Can you work these out from the model? Positions are in its coordinate system, mm. A direction names the side the tool comes from. Coordinates: 2 decimals unless noted, no trailing zeros. Write each loop counter-clockwise with the first axis right and the second up, starting at its lowest first coordinate (ties: lowest second). Pieces come first, ordered by that corner, then holes. Notation, with made-up numbers: M 80,-5.5 L 118,-5.5 A26 ccw 118,29.5 Z; hole C 40.5,85 d11. An arc over 180 degrees is marked long. Answer as a JSON object with one key per item and string values. Group by question number.
from build123d import *

# Parameters (mm, degrees)
SKETCH1_R                = 15
BOSS_EXTRUDE1_DEPTH      = 75
CUT_EXTRUDE1_DEPTH       = 52
CUT_EXTRUDE2_DEPTH       = 3.5
SKETCH9_R                = 10
CUT_EXTRUDE12_DEPTH      = 70
SKETCH17_W               = 7
SKETCH17_H               = 12
CUT_EXTRUDE19_DEPTH      = 15
SKETCH19_W               = 7
SKETCH19_H               = 12
CUT_EXTRUDE20_DEPTH      = 15
SKETCH20_R               = 7.5
CUT_EXTRUDE21_DEPTH      = 40
CUT_EXTRUDE25_DEPTH      = 152.492574075
CUT_EXTRUDE25_DEPTH_BACK = 55
SKETCH21_W               = 20
SKETCH21_H               = 7.639320226
CUT_EXTRUDE28_DEPTH      = 152.492574075
CUT_EXTRUDE28_DEPTH_BACK = 10
SKETCH24_R               = 15
SKETCH25_R               = 15
CUT_EXTRUDE29_DEPTH      = 10
CUT_EXTRUDE30_DEPTH      = 81.841883926
CUT_EXTRUDE30_DEPTH_BACK = 81.841883926


with BuildPart() as part:
    # Sketch1 → Boss-Extrude1 (new, symmetric)
    with BuildSketch(Plane(origin=(0, 0, 0), x_dir=(1, 0, 0), z_dir=(0, 1, 0))):
        with Locations(Location((0, 0, 0), (0, 0, 270))):
            Circle(SKETCH1_R)
    extrude(amount=BOSS_EXTRUDE1_DEPTH, both=True)

    # Sketch2 → Cut-Extrude1 (cut)
    with BuildSketch(Plane.XZ.offset(75)):
        with BuildLine():
            Line((3.5, 15), (3.5, -15))
            ThreePointArc((3.5, -15), (0, -18.5), (-3.5, -15))
            Line((-3.5, -15), (-3.5, 15))
            ThreePointArc((-3.5, 15), (0, 18.5), (3.5, 15))
        make_face()
    extrude(amount=-CUT_EXTRUDE1_DEPTH, mode=Mode.SUBTRACT)

    # Sketch3 → Cut-Extrude2 (cut, symmetric)
    with BuildSketch(Plane(origin=(0, -26.5, 0), x_dir=(1, 0, 0), z_dir=(0, 1, 0))):
        Polygon((-14.980069936, 0), (-15.328117643, -9.993941304), (-0.348047707, -16.993941304), (0, -7), align=None)
        Polygon((15, 0), (0, 7), (0.348047707, 16.993941304), (15.348047707, 9.993941304), align=None)
    extrude(amount=CUT_EXTRUDE2_DEPTH, both=True, mode=Mode.SUBTRACT)

    # Sketch9 → Cut-Extrude12 (cut)
    with BuildSketch(Plane.XZ.offset(75)):
        with Locations(Location((0, 0, 0), (0, 0, 270))):
            Circle(SKETCH9_R)
    extrude(amount=-CUT_EXTRUDE12_DEPTH, mode=Mode.SUBTRACT)

    # Sketch17 → Cut-Extrude19 (cut)
    with BuildSketch(Plane(origin=(15, 0, 0), x_dir=(0, 0, -1), z_dir=(1, 0, 0))):
        with Locations((3.5, -29)):
            Rectangle(SKETCH17_W, SKETCH17_H)
    extrude(amount=-CUT_EXTRUDE19_DEPTH, mode=Mode.SUBTRACT)

    # Sketch19 → Cut-Extrude20 (cut)
    with BuildSketch(Plane.ZY.offset(15)):
        with Locations((3.5, -29)):
            Rectangle(SKETCH19_W, SKETCH19_H)
    extrude(amount=-CUT_EXTRUDE20_DEPTH, mode=Mode.SUBTRACT)

    # Sketch20 → Cut-Extrude21 (cut)
    with BuildSketch(Plane(origin=(0, 75, 0), x_dir=(1, 0, 0), z_dir=(0, 1, 0))):
        with Locations(Location((0, 0, 0), (0, 0, 270))):
            Circle(SKETCH20_R)
    extrude(amount=-CUT_EXTRUDE21_DEPTH, mode=Mode.SUBTRACT)

    # Sketch21 → Cut-Extrude25 (cut, two sides: drawn at the far end of the back side and taken through both)
    with BuildSketch(Plane(origin=(0, 75, 0), x_dir=(1, 0, 0), z_dir=(0, 1, 0)).offset(-CUT_EXTRUDE25_DEPTH_BACK)):
        with Locations((0, 15)):
            Rectangle(SKETCH21_W, SKETCH21_H)
        with Locations((0, -15)):
            Rectangle(SKETCH21_W, SKETCH21_H)
    extrude(amount=CUT_EXTRUDE25_DEPTH + CUT_EXTRUDE25_DEPTH_BACK, mode=Mode.SUBTRACT)

    # Sketch24 → Cut-Extrude28 (cut, two sides: drawn at the far end of the back side and taken through both)
    with BuildSketch(Plane(origin=(0, 75, 0), x_dir=(1, 0, 0), z_dir=(0, 1, 0)).offset(-CUT_EXTRUDE28_DEPTH_BACK)):
        with Locations(Location((0, 0, 0), (0, 0, 76.506601178))):
            Circle(SKETCH24_R)
    extrude(amount=CUT_EXTRUDE28_DEPTH + CUT_EXTRUDE28_DEPTH_BACK, mode=Mode.SUBTRACT)

    # Sketch25 → Cut-Extrude29 (cut)
    with BuildSketch(Plane(origin=(0, 65, 0), x_dir=(1, 0, 0), z_dir=(0, 1, 0))):
        with Locations(Location((0, 0, 0), (0, 0, 76.506601178))):
            Circle(SKETCH25_R)
    extrude(amount=-CUT_EXTRUDE29_DEPTH, mode=Mode.SUBTRACT)

    # Sketch26 → Cut-Extrude30 (cut, two sides: drawn at the far end of the back side and taken through both)
    with BuildSketch(Plane.XY.offset(11.180339887).offset(-CUT_EXTRUDE30_DEPTH_BACK)):
        with BuildLine():
            Line((6, 45), (6, 35))
            ThreePointArc((6, 35), (0, 29), (-6, 35))
            Line((-6, 35), (-6, 45))
            ThreePointArc((-6, 45), (0, 51), (6, 45))
        make_face()
    extrude(amount=CUT_EXTRUDE30_DEPTH + CUT_EXTRUDE30_DEPTH_BACK, mode=Mode.SUBTRACT)


solid = part.part
Q1. If we section it at C-C on x = 0: List the corners of the cut face in (y, z) for me, and give its area (3 significant figures).
Q2. Please list where these lines run through material, in increasing order: L1, parallel to X at y = 46.5, z = 0; L2, parallel to X at y = -32.5, z = 10; L3, parallel to Y at x = 12.5, z = -3.5.
Q3. We'd pull the mould along Y, two halves only. Please class faces 1 (the flat face through (-10, -33, 7)), 2 (the flat face through (0, 20, -13)), 3 (the flat face through (0, -5, 0)), 4 (the flat face through (-7, 37, 11.18)): pulls with the +Y half, pulls with the -Y half, needs draft (parallel to the pull), parting line crosses it, or undercut.
Q4. If we section it at B-B on y = 38.5: List the corners of the cut face in (x, z) for me, and give its area (3 significant figures).
Q5. Will these pins go through, and if not, where does the flat tip stop? pin 1 (16 mm diameter, centred on x = -2, y = 30, fed in from -Z); pin 2 (1 mm diameter, centred on x = -9.5, y = -54.5, fed in from -Z); pin 3 (4 mm diameter, centred on y = -57.5, z = 11.5, fed in from +X); pin 4 (12 mm diameter, centred on x = 5.5, z = -5.5, fed in from -Y).
Q6. If we section it at A-A on y = -33: List the corners of the cut face in (x, z) for me, and give its area (3 significant figures).
Q7. On a 3-axis mill with a long thin cutter (end or side, diameter ignored), from which of +Z, -Z, +X, -X, +Y, -Y can I reach the whole of each face in a straight line? I mean faces 5 (the flat face through (7, -30, -10)), 6 (the cylindrical face through (-8.872, -40.49, -4.614)), 7 (the cylindrical face through (0, 51, -9)). Say none if no direction works.
Reply:
{
 "1": {"outline": "M -23,-15 L 20,-15 L 20,-11.18 L 29,-11.18 L 29,11.18 L 20,11.18 L 20,15 L -23,15 L -23,10 L -5,10 L -5,-10 L -23,-10 Z; M 51,-11.18 L 55,-11.18 L 55,-7.5 L 51,-7.5 Z; M 51,7.5 L 55,7.5 L 55,11.18 L 51,11.18 Z", "area": "1,160 mm^2"},
 "2": {"L1": "-15 to -7.5, 7.5 to 15", "L2": "-11.18 to -3.5, 3.5 to 11.18", "L3": "-75 to -35, -23 to 55"},
 "3": {"face 1": "undercut", "face 2": "pulls with the +Y half", "face 3": "pulls with the -Y half", "face 4": "needs draft"},
 "4": {"outline": "M -10,-11.18 L -6,-11.18 L -6,-4.5 A7.5 cw -6,4.5 L -6,11.18 L -10,11.18 A15 ccw Z; M 6,-11.18 L 10,-11.18 A15 ccw 10,11.18 L 6,11.18 L 6,4.5 A7.5 cw 6,-4.5 Z", "area": "315 mm^2"},
 "5": {"pin 1": "z = -11.18", "pin 2": "z = -12", "pin 3": "x = 11.61", "pin 4": "y = -75"},
 "6": {"outline": "M -15,0 A15 ccw -3.5,-14.59 L -3.5,-9.37 A10 cw -10,0 Z; M -13.27,7 L -7.14,7 A10 cw -3.5,9.37 L -3.5,14.59 A15 ccw Z; M 3.5,-14.59 A15 ccw 13.27,-7 L 7.14,-7 A10 cw 3.5,-9.37 Z; M 3.5,9.37 A10 cw 10,0 L 15,0 A15 ccw 3.5,14.59 Z", "area": "247 mm^2"},
 "7": {"face 5": "-Z, +X", "face 6": "-Y", "face 7": "+Z, -Z"}
}
